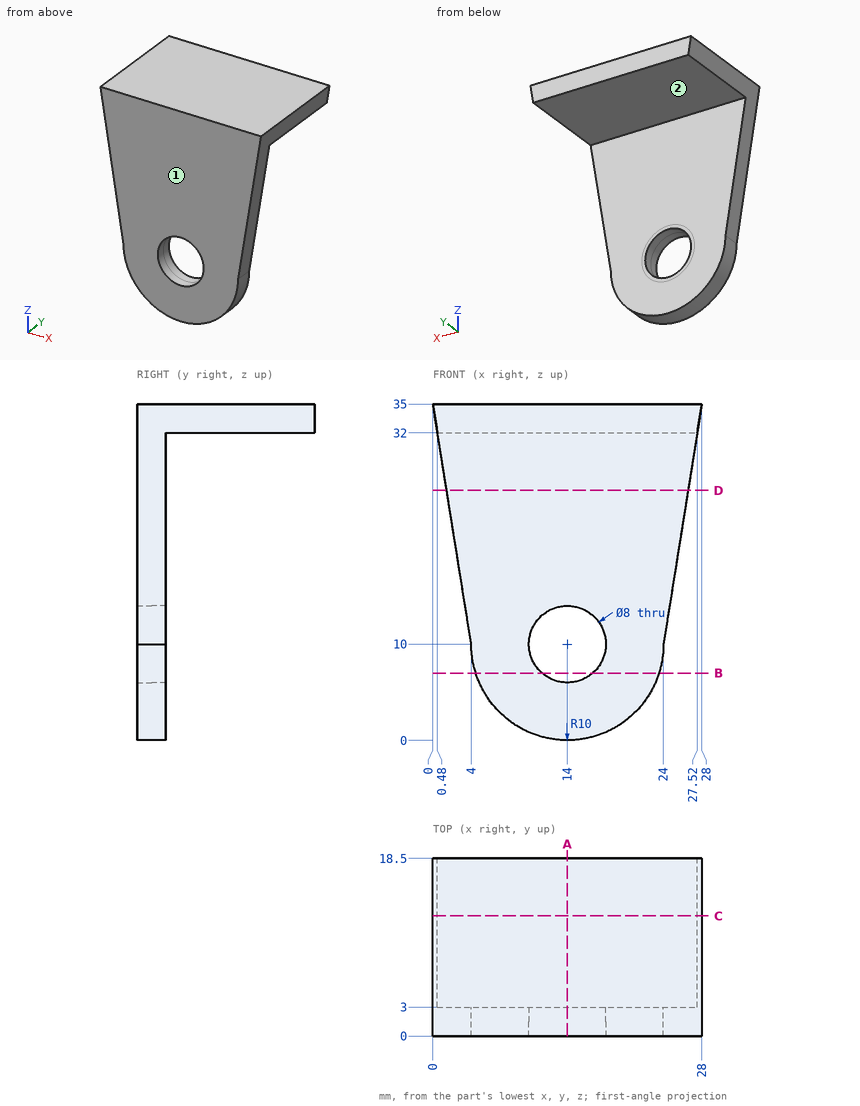
The figure shows three views and two pictorial views of one solid part (mm, origin at its lowest corner). Answer the questions. A direction names the side the tool comes from. Give positions to 0.01 mm unless a question says otherwise; leave off trailing zeros. Write each loop counter-clockwise with the first axis right and the second up, starting at its lowest first coordinate (ties: lowest second). Pieces come first, ordered by that corner, then holes. Notation, with made-up numbers: (23, -34.75) - (67, -34.75) arc R6 ccw to (67, -30.75) - close; hole circle Ø4 at (47, -36). An arc over 180 degrees is marked (long way). Return JSON: item names as keys, results as strings.
Q1. For the marked faces 1 and 2, determine the directions among +Z, -Z, +X, -X, +Y, -Y from which every point of the face is accessible in a straight line to the end or side of a thin tool.
Reply:
{"face 1": "+Z, -Z, +X, -X, -Y", "face 2": "-Z, +X, -X, +Y"}
Q2. A cutting plane is placed at C-C, the plane y = 12.5. Determine the outline of the cut face in (x, z).
Reply:
{"outline": "(0, 35) - (0.48, 32) - (27.52, 32) - (28, 35) - close"}
Q3. A cutting plane is placed at D-D, the plane z = 26. Determine the outline of the cut face in (x, y), and give its area (3 significant figures).
Reply:
{"outline": "(1.44, 0) - (26.56, 0) - (26.56, 3) - (1.44, 3) - close", "area": "75.4 mm²"}
Q4. Given P1, Ø8, axis at x = 19.5, y = 8, coming from the -Z side; P2, Ø7, axis at x = 14, z = 10, coming from the +Y side; P3, Ø3, axis at x = 14.5, z = 16, coming from the +Y side, each flat-ended and moving along its own axis, determine where each tip first touches the part or whether it passes through.
Reply:
{"P1": "z = 32", "P2": "through", "P3": "y = 3"}
Q5. A cutting plane is placed at B-B, the plane z = 7. Determine the outline of the cut face in (x, y).
Reply:
{"outline": "(4.46, 0) - (11.35, 0) - (11.35, 3) - (4.46, 3) - close; (16.65, 0) - (23.54, 0) - (23.54, 3) - (16.65, 3) - close"}
Q6. Consider line 1 along Z through (x, y) = (14, 0.6); line 2 along X through (y, z) = (2.5, 10); line 3 along Z through (x, y) = (14, 8.5). Determine where each line is inside the solid, lowest interval first. Write a range as [from, to].
Reply:
{"line 1": "[0, 6], [14, 35]", "line 2": "[4, 10], [18, 24]", "line 3": "[32, 35]"}
Q7. A cutting plane is placed at A-A, the plane x = 14. Determine the outline of the cut face in (y, z).
Reply:
{"outline": "(0, 0) - (3, 0) - (3, 6) - (0, 6) - close; (0, 14) - (3, 14) - (3, 32) - (18.5, 32) - (18.5, 35) - (0, 35) - close"}
